Solid Edge part; units mm, degrees
sketch "Sketch1" plane through (0, 0, 0) normal (0, -1, 0) x (1, 0, 0)
  line L0 (4.5, 18.5) -> (4.5, 22.5)
  line L1 (4.5, 22.5) -> (0, 22.5)
  line L2 (0, 22.5) -> (0, 0)
  line L3 (0, 0) -> (4.5, 0)
  line L4 (4.5, 0) -> (4.5, 1.5)
  line L5 (4.5, 1.5) -> (6, 1.5)
  line L6 (6, 1.5) -> (6, 2.5)
  line L7 (6, 2.5) -> (4.5, 2.5)
  line L8 (4.5, 2.5) -> (4.5, 15.5)
  line L9 (4.5, 15.5) -> (3, 15.5)
  line L10 (3, 15.5) -> (3, 18.5)
  line L11 (3, 18.5) -> (4.5, 18.5)
revolve "RevolvedProtrusion1" add sketch "Sketch1" angle 360 about axis through (0, 0, 22.5) along (0, 0, -1)
fillet "Round1" radius 1.5 3 edges at (-3, 0, 15.5) (-4.5, 0, 2.5) (-4.5, 0, 1.5)
fillet "Round_2" radius 2 1 edges at (-4.5, 0, 22.5)
sketch "Sketch2" plane through (0, 0, 0) normal (0, 0, -1) x (1, 0, 0)
  circle A0 centre (0, 0) radius 4.5
extrude "ProtrusiónExtruida_1" add sketch "Sketch2" along normal blind 22
Work out the finished part from the listing and answer in its coordinate system (mm). A direction names the side the tool comes from. Round coordinates to 2 decimals unless told otherwise and drop trailing zeros. Loops run counter-clockwise (first coordinate to the right, second up) from the corner with the lowest first, then second, coordinate; pieces in that order, holes last.
(1) The mould has two halves that part along Z. Classify faces 6 (the flat face through (0, 0, 22.5)), 7 (the flat face through (1, 3, 18.5)), 8 (the cylindrical face through (-0.59, 4.46, 19.51)): pulls with the +Z half, pulls with the -Z half, needs draft (parallel to the pull), parting line crosses it, or undercut.
Computed values:
face 6: pulls with the +Z half
face 7: undercut
face 8: needs draft
(2) Each of these flat-tipped pins is pushed along its axis until it touches: P1, Ø1.5, axis at y = -0.5, z = -11.5, coming from the +X side; P2, Ø4, axis at y = 0, z = 3.5, coming from the +X side; P3, Ø1.5, axis at y = -2, z = -16, coming from the -X side; P4, Ø1.5, axis at y = -4.5, z = -15.5, coming from the +X side. Where does it stop, or does it pass through?
Computed values:
P1: stops at x = 4.5
P2: stops at x = 6
P3: stops at x = -4.32
P4: stops at x = 2.49
(3) The part is cut by section C-C, the plane z = 6. Give the vertices of the cut face in (x, y), and give its area (3 significant figures).
Computed values:
outline: circle Ø9 at (0, 0)
area: 63.6 mm2
(4) Find the intervals of material crossed by L1, parallel to Z at x = -2.5, y = 0.75; L2, parallel to Z at x = 1.25, y = 3.5; L3, parallel to Y at x = -1, z = -12, in increasing order.
Computed values:
L1: z = -22 to 22.5
L2: z = -22 to 15.72, 18.5 to 22.09
L3: y = -4.39 to 4.39
(5) For faces 1 (the flat face through (0, 0, -22)), 2 (the cylindrical face through (-3, 0, 18)), 3 (the cylindrical face through (-0.59, 4.46, 9.83)), 4 (the cylindrical face through (-0.59, 4.46, -10.85)), 5 (the cylindrical face through (-6, 0, 2)), determine the directions among +Z, -Z, +X, -X, +Y, -Y from which every point of the face is accessible in a straight line to the end or side of a thin tool.
Computed values:
face 1: -Z, +X, -X, +Y, -Y
face 2: none
face 3: +Z
face 4: -Z
face 5: +Z, -Z
